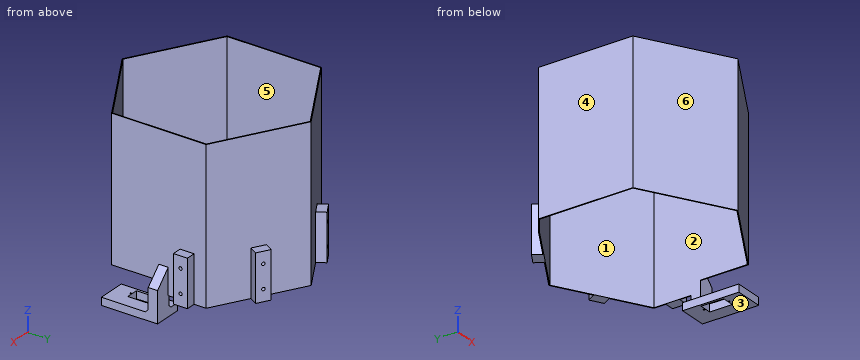
```python
from build123d import *

# Parameters (mm, degrees)
PAD_DEPTH       = 150
SKETCH001_W     = 17
SKETCH001_H     = 10
PAD001_DEPTH    = 25
SKETCH002_W     = 30
SKETCH002_H     = 60
PAD002_DEPTH    = 8
SKETCH003_W     = 13
SKETCH003_H     = 24
POCKET_DEPTH    = 8.001
SKETCH004_R     = 0.8
HOLE_DEPTH      = 25
CHAMFER_SIZE    = 16
CHAMFER001_SIZE = 3
PAD003_DEPTH    = 12
SKETCH006_W     = 15
SKETCH006_H     = 50
PAD004_DEPTH    = 10
SKETCH007_R     = 1.7
HOLE001_DEPTH   = 6
HOLE001_TIPS_R  = 1.7
SKETCH008_W     = 15
SKETCH008_H     = 50
PAD005_DEPTH    = 10
SKETCH009_R     = 1.7
HOLE002_DEPTH   = 6
HOLE002_TIPS_R  = 1.7
SKETCH010_W     = 15
SKETCH010_H     = 50
PAD006_DEPTH    = 10
SKETCH011_R     = 1.7
HOLE003_DEPTH   = 6
HOLE003_TIPS_R  = 1.7


with BuildPart() as part:
    # Sketch → Pad (new body)
    with BuildSketch(Plane.XY):
        Polygon((87.4685657822, -50.5), (87.4685657822, 50.5), (0, 101), (-87.4685657822, 50.5), (-87.4685657822, -50.5), (0, -101), align=None)
        Polygon((86.6025403784, 50), (0, 100), (-86.6025403784, 50), (-86.6025403784, -50), (0, -100), (86.6025403784, -50), align=None, mode=Mode.SUBTRACT)
    extrude(amount=PAD_DEPTH)

    # Sketch001 (on Face13 of Pad) → Pad001 (join)
    with BuildSketch(Plane(origin=(0, 0, 0), x_dir=(1, 0, 0), z_dir=(0, 0, -1))):
        with Locations((95.1025403784, -5)):
            Rectangle(SKETCH001_W, SKETCH001_H)
    extrude(amount=PAD001_DEPTH)

    # Sketch002 (on Face20 of Pad001) → Pad002 (join)
    with BuildSketch(Plane(origin=(0, 0, -25), x_dir=(1, 0, 0), z_dir=(0, 0, -1))):
        with Locations((88.6025403784, 20)):
            Rectangle(SKETCH002_W, SKETCH002_H)
    extrude(amount=PAD002_DEPTH)

    # Sketch003 (on Face21 of Pad002) → Pocket (cut, through all)
    with BuildSketch(Plane.XY.offset(-25)):
        with Locations((82.6025403784, -20)):
            Rectangle(SKETCH003_W, SKETCH003_H)
    extrude(amount=-POCKET_DEPTH, mode=Mode.SUBTRACT)

    # Sketch004 (on Face21 of Pocket) → Hole (cut)
    with BuildSketch(Plane.XY.offset(-25)):
        with Locations((82.6025403784, -6.379604)):
            Circle(SKETCH004_R)
        with Locations((82.6025403784, -33.379604)):
            Circle(SKETCH004_R)
    extrude(amount=-HOLE_DEPTH, mode=Mode.SUBTRACT)

    # Chamfer
    chamfer_edges = [part.edges().sort_by_distance(p)[0] for p in [
        (87.468566, 5, 0),
    ]]
    chamfer(chamfer_edges, length=CHAMFER_SIZE)

    # Chamfer001
    chamfer001_edges = [part.edges().sort_by_distance(p)[0] for p in [
        (95.10254, 0, -25),
        (86.60254, 5, -25),
    ]]
    chamfer(chamfer001_edges, length=CHAMFER001_SIZE)

    # Sketch005 (on Face7 of Chamfer001) → Pad003 (join)
    with BuildSketch(Plane(origin=(0, 0, 0), x_dir=(1, 0, 0), z_dir=(0, 0, -1))):
        Polygon((86.6025403784, -10), (86.6025403784, -50), (0, -100), (-86.6025403784, -50), (-87.4685657822, -50.5), (0, -101), (87.4685657822, -50.5), (87.4685657822, -10), align=None)
    extrude(amount=PAD003_DEPTH)

    # Sketch006 (on Face23 of Pad003) → Pad004 (join)
    with BuildSketch(Plane.YZ.offset(87.4685657822)):
        with Locations((30.25, 13)):
            Rectangle(SKETCH006_W, SKETCH006_H)
    extrude(amount=PAD004_DEPTH)

    # Sketch007 (on Face47 of Pad004) → Hole001 (cut)
    with BuildSketch(Plane.YZ.offset(97.4685657822)):
        with Locations((30.25, 25.5)):
            Circle(SKETCH007_R)
        with Locations((30.25, 0.5)):
            Circle(SKETCH007_R)
    extrude(amount=-HOLE001_DEPTH, mode=Mode.SUBTRACT)

    # Hole001 tips → Hole001 tip 1 section 0
    with BuildSketch(Plane.YZ.offset(91.4685657822), mode=Mode.PRIVATE) as hole001_tip_1_s0:
        with Locations((30.25, 25.5)):
            Circle(HOLE001_TIPS_R)
    loft([hole001_tip_1_s0.sketch, Vertex(90.4471027299, 30.25, 25.5)], mode=Mode.SUBTRACT)

    # Hole001 tips → Hole001 tip 2 section 0
    with BuildSketch(Plane.YZ.offset(91.4685657822), mode=Mode.PRIVATE) as hole001_tip_2_s0:
        with Locations((30.25, 0.5)):
            Circle(HOLE001_TIPS_R)
    loft([hole001_tip_2_s0.sketch, Vertex(90.4471027299, 30.25, 0.5)], mode=Mode.SUBTRACT)

    # Sketch008 (on Face48 of Hole001) → Pad005 (join)
    with BuildSketch(Plane(origin=(43.7342828911, 75.75, 0), x_dir=(-0.8660254038, 0.5, 0), z_dir=(0.5, 0.8660254038, 0))):
        with Locations((0, 13)):
            Rectangle(SKETCH008_W, SKETCH008_H)
    extrude(amount=PAD005_DEPTH)

    # Sketch009 (on Face56 of Pad005) → Hole002 (cut)
    with BuildSketch(Plane(origin=(48.7342828911, 84.4102540378, 0), x_dir=(-0.8660254038, 0.5, 0), z_dir=(0.5, 0.8660254038, 0))):
        with Locations((0, 25.5)):
            Circle(SKETCH009_R)
        with Locations((0, 0.5)):
            Circle(SKETCH009_R)
    extrude(amount=-HOLE002_DEPTH, mode=Mode.SUBTRACT)

    # Hole002 tips → Hole002 tip 1 section 0
    with BuildSketch(Plane(origin=(45.7342828911, 79.2141016151, 0), x_dir=(-0.8660254038, 0.5, 0), z_dir=(0.5, 0.8660254038, 0)), mode=Mode.PRIVATE) as hole002_tip_1_s0:
        with Locations((0, 25.5)):
            Circle(HOLE002_TIPS_R)
    loft([hole002_tip_1_s0.sketch, Vertex(45.2235513649, 78.3294886628, 25.5)], mode=Mode.SUBTRACT)

    # Hole002 tips → Hole002 tip 2 section 0
    with BuildSketch(Plane(origin=(45.7342828911, 79.2141016151, 0), x_dir=(-0.8660254038, 0.5, 0), z_dir=(0.5, 0.8660254038, 0)), mode=Mode.PRIVATE) as hole002_tip_2_s0:
        with Locations((0, 0.5)):
            Circle(HOLE002_TIPS_R)
    loft([hole002_tip_2_s0.sketch, Vertex(45.2235513649, 78.3294886628, 0.5)], mode=Mode.SUBTRACT)

    # Sketch010 (on Face44 of Hole002) → Pad006 (join)
    with BuildSketch(Plane(origin=(-43.7342828911, 75.75, 0), x_dir=(-0.8660254038, -0.5, 0), z_dir=(-0.5, 0.8660254038, 0))):
        with Locations((0, 13)):
            Rectangle(SKETCH010_W, SKETCH010_H)
    extrude(amount=PAD006_DEPTH)

    # Sketch011 (on Face62 of Pad006) → Hole003 (cut)
    with BuildSketch(Plane(origin=(-48.7342828911, 84.4102540378, 0), x_dir=(-0.8660254038, -0.5, 0), z_dir=(-0.5, 0.8660254038, 0))):
        with Locations((0, 25.5)):
            Circle(SKETCH011_R)
        with Locations((0, 0.5)):
            Circle(SKETCH011_R)
    extrude(amount=-HOLE003_DEPTH, mode=Mode.SUBTRACT)

    # Hole003 tips → Hole003 tip 1 section 0
    with BuildSketch(Plane(origin=(-45.7342828911, 79.2141016151, 0), x_dir=(-0.8660254038, -0.5, 0), z_dir=(-0.5, 0.8660254038, 0)), mode=Mode.PRIVATE) as hole003_tip_1_s0:
        with Locations((0, 25.5)):
            Circle(HOLE003_TIPS_R)
    loft([hole003_tip_1_s0.sketch, Vertex(-45.2235513649, 78.3294886628, 25.5)], mode=Mode.SUBTRACT)

    # Hole003 tips → Hole003 tip 2 section 0
    with BuildSketch(Plane(origin=(-45.7342828911, 79.2141016151, 0), x_dir=(-0.8660254038, -0.5, 0), z_dir=(-0.5, 0.8660254038, 0)), mode=Mode.PRIVATE) as hole003_tip_2_s0:
        with Locations((0, 0.5)):
            Circle(HOLE003_TIPS_R)
    loft([hole003_tip_2_s0.sketch, Vertex(-45.2235513649, 78.3294886628, 0.5)], mode=Mode.SUBTRACT)


solid = part.part
```
Geometry: final body of the model. Coordinates: model frame, mm. Face numbers are marked on the shaded views. A direction names the side the tool comes from. Give positions to 0.01 mm unless a question says otherwise; leave off trailing zeros. Order: outer loops, then holes, each group sorted by start corner. A loop starts at its lowest first (then second) coordinate and runs counter-clockwise, first axis right, second up. Notation, with made-up numbers: (86.25, 49.5) -> (122.25, 49.5) arc R30 cw to (122.25, 84.5) -> close; hole circle Ø7 at (-4.5, 54.25). An arc over 180 degrees is marked (long way). Write each question's results on one line, items separated by ' | '. Start each with the question number.
1) Line query: line 1 (Z direction, x = 93.1, y = 30.25); line 2 (X direction, y = -32.5, z = 136); line 3 (Y direction, x = 73.5, z = 17). Output: solid intervals per line, ascending. Write a range as from..to.
2) Section C-C (x = -58). Return loops of the section in (y, z), then the cut area to 3 significant figures.
3) Section D-D (y = 55). Return loops of the section in (x, z).
4) Section B-B (z = 75.5). Return loops of the section in (x, y), then the cut area to 3 significant figures.
5) First-contact query: pin 1 (9 mm diameter, centred on x = 81.5, z = -29.5, fed in from -Y); pin 2 (12 mm diameter, centred on x = -50, z = 60, fed in from +Y); pin 3 (2 mm diameter, centred on x = -27.5, z = -10, fed in from +Y). Flat tips, straight axial feed; report the tip coordinate or a pass-through.
6) Draft query along Y for the marked faces 4, 5 and 6. Return one class per face: pulls with the +Y half, pulls with the -Y half, needs draft (parallel to the pull), parting line crosses it, or undercut.
7) Section A-A (y = -26). Return loops of the section in (x, z).
8) Set-up query: the marked faces 1, 2 and 3. Return all of +Z, -Z, +X, -X, +Y, -Y with unobstructed straight access to the full face (end or side cutting, diameter ignored); none if empty.
Calculated:
1) line 1: -12..-1.2, 2.2..23.8, 27.2..38 | line 2: -87.47..-86.6, 86.6..87.47 | line 3: -58.56..-57.56, 57.56..58.56
2) outline: (-67.51, 0) -> (-66.51, 0) -> (-66.51, 150) -> (-67.51, 150) -> close; (66.51, -12) -> (67.51, -12) -> (67.51, 150) -> (66.51, 150) -> close | area: 312 mm2
3) outline: (-79.67, -12) -> (-77.94, -12) -> (-77.94, 150) -> (-79.67, 150) -> close; (77.94, -12) -> (79.67, -12) -> (79.67, 150) -> (77.94, 150) -> close
4) outline: (-87.47, -50.5) -> (0, -101) -> (87.47, -50.5) -> (87.47, 50.5) -> (0, 101) -> (-87.47, 50.5) -> close; hole (-86.6, -50) -> (0, -100) -> (86.6, -50) -> (86.6, 50) -> (0, 100) -> (-86.6, 50) -> close | area: 522 mm2
5) pin 1: y = -50 | pin 2: y = 75.6 | pin 3: y = 85.7
6) face 4: needs draft | face 5: undercut | face 6: pulls with the -Y half
7) outline: (-87.47, 0) -> (-86.6, 0) -> (-86.6, 150) -> (-87.47, 150) -> close; (73.6, -33) -> (76.1, -33) -> (76.1, -25) -> (73.6, -25) -> close; (86.6, 0) -> (87.47, 0) -> (87.47, 150) -> (86.6, 150) -> close; (89.1, -33) -> (103.6, -33) -> (103.6, -25) -> (89.1, -25) -> close
8) face 1: +Z, -Z | face 2: +Z | face 3: -Z, +X, -X, +Y, -Y
